```python
from build123d import *

# Parameters (mm, degrees)
BOSS_EXTRUDE1_DEPTH   = 3.175
FILLET1_R             = 6.35
F_2_56_TAPPED_HOLE2_D = 1.778
CUT_EXTRUDE1_DEPTH    = 75.069947742
FILLET2_R             = 1.5875


with BuildPart() as part:
    # Sketch1 → Boss-Extrude1 (new body)
    with BuildSketch(Plane.XY):
        with BuildLine():
            Line((-4.835969239, 0), (18.250637604, -39.987176027))
            ThreePointArc((18.250637604, -39.987176027), (23.298677844, -40.879278308), (25.623151786, -36.310320261))
            Line((25.623151786, -36.310320261), (8.49045675, 65.376366097))
            ThreePointArc((8.49045675, 65.376366097), (3.466101861, 69.394963614), (-1.090256537, 64.852622125))
            Line((-1.090256537, 64.852622125), (-4.835969239, 0))
        make_face()
    extrude(amount=BOSS_EXTRUDE1_DEPTH)

    # Fillet1
    fillet1_edges = [part.edges().sort_by_distance(p)[0] for p in [
        (-4.835969239, 0, 1.5875),
    ]]
    fillet(fillet1_edges, radius=FILLET1_R)

    # #2-56 Tapped Hole2 (through all)
    with Locations(Plane(origin=(2.631187962, 45.555933465, 3.175), x_dir=(1, 0, 0), z_dir=(0, 0, 1))):
        with Locations((0, 0), (0.732297358, 12.678869847), (1.098446037, 19.01830477)):
            Hole(F_2_56_TAPPED_HOLE2_D / 2)

    # Sketch5 → Cut-Extrude1 (cut, through all)
    with BuildSketch(Plane.XY.offset(3.175)):
        Polygon((2.537667609, 43.936738235), (7.314221402, 43.936738235), (10.071596328, 28.061738235), (1.620770386, 28.061738235), align=None)
        Polygon((1.437390941, 24.886738235), (10.623071313, 24.886738235), (12.277496268, 15.361738235), (0.887252607, 15.361738235), align=None)
        Polygon((0.703873162, 12.186738235), (12.828971253, 12.186738235), (14.669983772, 1.5875), (0.091689722, 1.5875), align=None)
        Polygon((0.916543552, -1.5875), (15.221458757, -1.5875), (16.875883712, -11.1125), (6.415804866, -11.1125), align=None)
        Polygon((21.376833522, -37.025761765), (17.427358698, -14.2875), (8.248891971, -14.2875), align=None)
    extrude(amount=-CUT_EXTRUDE1_DEPTH, mode=Mode.SUBTRACT)

    # Fillet2
    fillet2_edges = [part.edges().sort_by_distance(p)[0] for p in [
        (1.620770386, 28.061738235, 1.5875),
        (2.537667609, 43.936738235, 1.5875),
        (7.314221402, 43.936738235, 1.5875),
        (10.071596328, 28.061738235, 1.5875),
        (6.415804866, -11.1125, 1.5875),
        (0.916543552, -1.5875, 1.5875),
        (15.221458757, -1.5875, 1.5875),
        (16.875883712, -11.1125, 1.5875),
        (0.091689722, 1.5875, 1.5875),
        (0.703873162, 12.186738235, 1.5875),
        (12.828971253, 12.186738235, 1.5875),
        (14.669983772, 1.5875, 1.5875),
        (0.887252607, 15.361738235, 1.5875),
        (1.437390941, 24.886738235, 1.5875),
        (10.623071313, 24.886738235, 1.5875),
        (12.277496268, 15.361738235, 1.5875),
        (21.376833522, -37.025761765, 1.5875),
        (8.248891971, -14.2875, 1.5875),
        (17.427358698, -14.2875, 1.5875),
    ]]
    fillet(fillet2_edges, radius=FILLET2_R)


solid = part.part
```
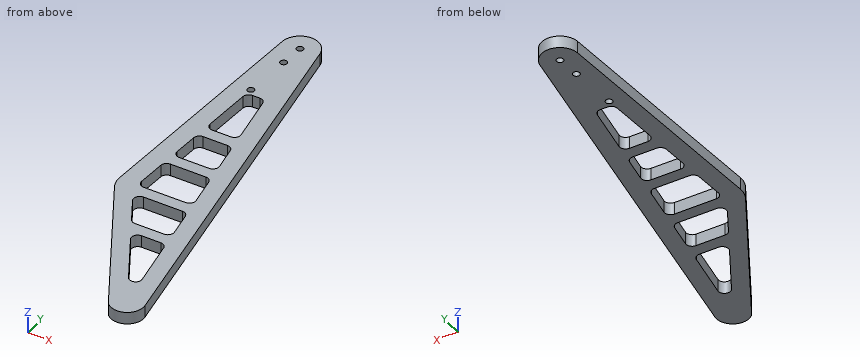
The model under review builds one solid part; all positions refer to its coordinate system, in mm. Coordinates: 2 decimals unless noted, no trailing zeros. Order: outer loops, then holes, each group sorted by start corner. A loop starts at its lowest first (then second) coordinate and runs counter-clockwise, first axis right, second up. Notation, with made-up numbers: (39.5, -29) -> (64.5, -29) arc R28 ccw to (64.5, -10) -> close; hole circle Ø1 at (79, 49). An arc over 180 degrees is marked (long way). Answer in a Markdown table with one row per item. Add a question column.
Item 1: To check wall thickness, follow probe 1 along Y at (x, z) = (7, 2.8); probe 2 along Y at (x, z) = (6.5, 1.45); probe 3 along X at (y, z) = (23.5, 0.7). State the ranges of each line that lie inside material, in increasing order.
Item 2: Clearance check with flat-ended pins moving along their axes: pin 1 (1.6 mm diameter, centred on x = 5, z = 2, fed in from +Y); pin 2 (1.6 mm diameter, centred on x = 5.5, z = 2, fed in from -Y); pin 3 (1 mm diameter, centred on x = 5, z = 2, fed in from -Y). State where each tip first meets the part, or that it passes through.
Item 3: We need section C-C on y = 48.5. Write out the cut boundary in (x, z) (3 decimals), plus the area to 3 significant figures.
Item 4: We need section A-A on y = 9. Write out the cut boundary in (x, z) (3 decimals).
Item 5: We need section B-B on z = 2.15. Give the number of separate pieces and of enclosed holes in the cut face, plus the area to 3 significant figures.
Final values:
| question | item | result |
|---|---|---|
| 1 | probe 1 | y = -20.5 to -11.08, -1.59 to 1.59, 12.19 to 15.36, 24.89 to 28.06, 43.56 to 68.13 |
| 1 | probe 2 | y = -19.63 to -10.88, -1.59 to 1.59, 12.19 to 15.36, 24.89 to 28.06, 43.85 to 68.53 |
| 1 | probe 3 | x = -3.48 to 1.36, 10.86 to 15.55 |
| 2 | pin 1 | stops at y = 69.38 |
| 2 | pin 2 | stops at y = -19.29 |
| 2 | pin 3 | stops at y = -17.9 |
| 3 | outline | (-2.035, 0) -> (11.334, 0) -> (11.334, 3.175) -> (-2.035, 3.175) -> close |
| 3 | area | 42.4 mm2 |
| 4 | outline | (-4.316, 0) -> (0.52, 0) -> (0.52, 3.175) -> (-4.316, 3.175) -> close; (13.382, 0) -> (17.989, 0) -> (17.989, 3.175) -> (13.382, 3.175) -> close |
| 5 | separate pieces | 1 |
| 5 | enclosed holes | 8 |
| 5 | area | 1,230 mm2 |
